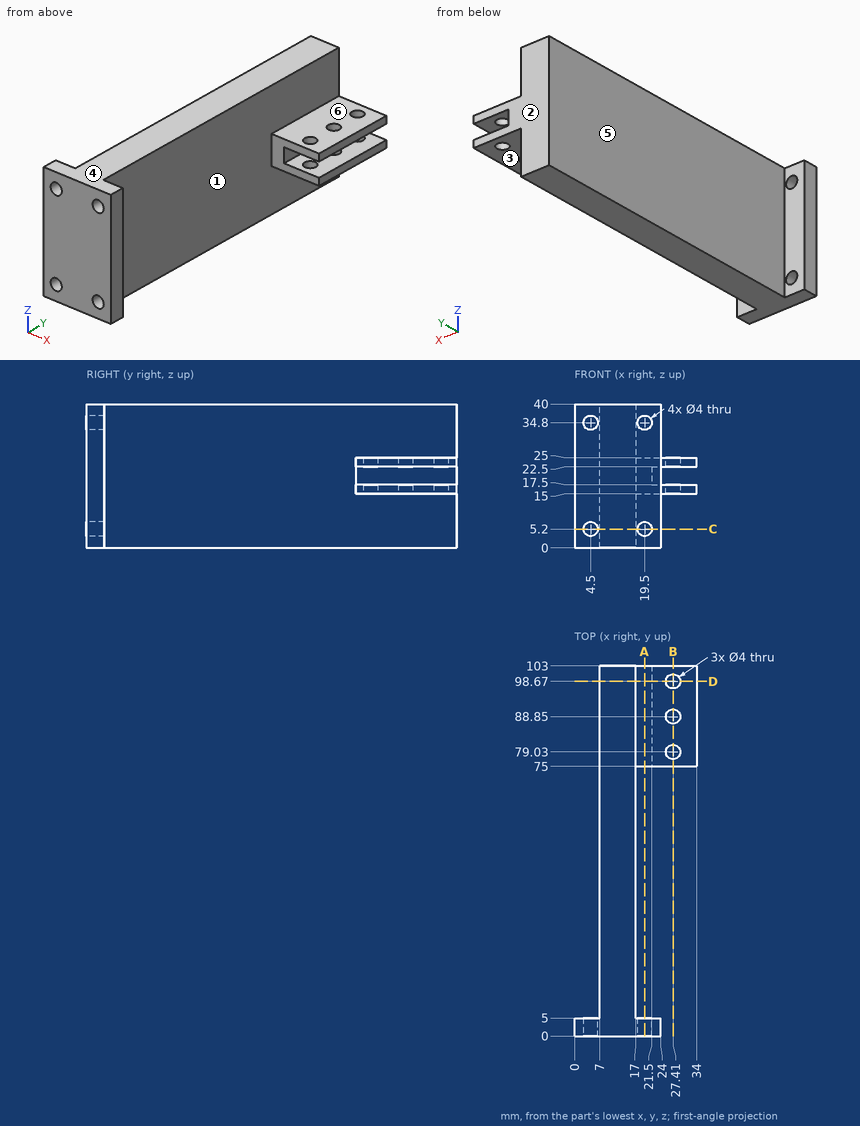
Verification items for this drawing (mm, ordinates from the low corner). A direction names the side the tool comes from. Give positions to 0.01 mm unless a question says otherwise; leave off trailing zeros. Loops run counter-clockwise (first coordinate to the right, second up) from the corner with the lowest first, then second, coordinate; pieces in that order, holes last. Notation, with made-up numbers: M 25.25,82.25 L 58.25,82.25 A19 cw 58.25,109.25 Z; hole C 70.5,27.25 d10. An arc over 180 degrees is marked long. Return JSON: item names as keys, results as strings. Group by question number.
1. Thickness scan on L1, parallel to Y at x = 27.41, z = 24.45; L2, parallel to Z at x = 19.5, y = 2.8; L3, parallel to X at y = 3.9, z = 5.2. Record the ranges inside material, lowest first.
2. Cross-section at C-C on z = 5.2. Record the boundary of the cut face in (x, y), plus the area to 3 significant figures.
3. Tool access check on the marked faces 4, 5 and 6. Record the directions out of +Z, -Z, +X, -X, +Y, -Y that give a thin tool (end or side, any length) a straight path to the whole face; none if there is none.
4. Go/stop test with flat-tipped pins: pin 1 (12 mm diameter, centred on y = 59, z = 25.5, fed in from -X); pin 2 (8 mm diameter, centred on y = 30, z = 28, fed in from +X); pin 3 (4 mm diameter, centred on x = 21.5, z = 8.5, fed in from +Y). Record where each tip stops, or that it passes through.
5. Cross-section at B-B on x = 27.41. State how many separate pieces and enclosed holes the cut face has, plus the area to 3 significant figures.
6. Mould release check, pull along Y, two halves, no side actions. Record for the marked faces 1, 2 and 3: released by +Y, released by -Y, zero draft, split by the parting line, or undercut.
7. Cross-section at A-A on x = 19.5. Record the boundary of the cut face in (y, z).
8. Cross-section at D-D on y = 98.67. Record the boundary of the cut face in (x, z).
Return value:
{
 "1": {"L1": "75 to 77.03, 81.03 to 86.85, 90.85 to 96.67, 100.67 to 103", "L2": "0 to 3.2, 7.2 to 32.8, 36.8 to 40", "L3": "0 to 2.5, 6.5 to 17.5, 21.5 to 24"},
 "2": {"outline": "M 0,0 L 2.5,0 L 2.5,5 L 0,5 Z; M 6.5,0 L 17.5,0 L 17.5,5 L 17,5 L 17,103 L 7,103 L 7,5 L 6.5,5 Z; M 21.5,0 L 24,0 L 24,5 L 21.5,5 Z", "area": "1,060 mm^2"},
 "3": {"face 4": "+Z, +X, -X, +Y, -Y", "face 5": "+Z, -Z, -X, +Y", "face 6": "+Z, +X, +Y"},
 "4": {"pin 1": "x = 7", "pin 2": "x = 17", "pin 3": "y = 5"},
 "5": {"separate pieces": "8", "enclosed holes": "0", "area": "80.0 mm^2"},
 "6": {"face 1": "undercut", "face 2": "released by +Y", "face 3": "zero draft"},
 "7": {"outline": "M 0,0 L 5,0 L 5,3.2 L 0,3.2 Z; M 0,7.2 L 5,7.2 L 5,32.8 L 0,32.8 Z; M 0,36.8 L 5,36.8 L 5,40 L 0,40 Z; M 75,15 L 103,15 L 103,25 L 75,25 Z"},
 "8": {"outline": "M 7,0 L 17,0 L 17,15 L 25.41,15 L 25.41,17.5 L 21.5,17.5 L 21.5,22.5 L 25.41,22.5 L 25.41,25 L 17,25 L 17,40 L 7,40 Z; M 29.41,15 L 34,15 L 34,17.5 L 29.41,17.5 Z; M 29.41,22.5 L 34,22.5 L 34,25 L 29.41,25 Z"}
}
